```python
from build123d import *

# Parameters (mm, degrees)
SKETCH_1_R          = 4
EXTRUDE_1_DEPTH     = 3
EXTRUDE_2_DEPTH     = 3
SKETCH_3_W          = 36.5
SKETCH_3_H          = 5.8
SKETCH_3_R          = 0.65
EXTRUDE_3_DEPTH     = 1.75
SKETCH_3_4_R        = 1
CUT_EXTRUDE_1_DEPTH = 1.2
EXTRUDE_START       = -22
SKETCH_3_5_W        = 36.5
SKETCH_3_5_H        = 5.8
SKETCH_3_5_R        = 0.65
EXTRUDE_4_DEPTH     = 1.75
CUT_EXTRUDE_START   = -20.8
SKETCH_3_6_R        = 1
CUT_EXTRUDE_2_DEPTH = 1.2
SKETCH_5_R          = 0.4
CUT_EXTRUDE_3_DEPTH = 2


with BuildPart() as part:
    # 草图1 → 凸台-拉伸1 (new body)
    with BuildSketch(Plane(origin=(0, 0, 0), x_dir=(0, 0, -1), z_dir=(1, 0, 0))):
        with BuildLine():
            ThreePointArc((-13.5, 3.1e-08), (-11.998004256, -6.188529216), (-7.826237921, -11))
            Line((-7.826237921, -11), (7.826237921, -11))
            ThreePointArc((7.826237921, -11), (11.998004249, -6.18852923), (13.5, 0))
            ThreePointArc((13.5, 0), (11.998004249, 6.18852923), (7.826237921, 11))
            Line((7.826237921, 11), (-7.826237921, 11))
            ThreePointArc((-7.826237921, 11), (-11.998004242, 6.188529244), (-13.5, 3.1e-08))
        make_face()
        Circle(SKETCH_1_R, mode=Mode.SUBTRACT)
    extrude(amount=EXTRUDE_1_DEPTH)

    # 草图2 → 凸台-拉伸2 (add)
    with BuildSketch(Plane(origin=(3, 0, 0), x_dir=(0, 0, -1), z_dir=(1, 0, 0))):
        with BuildLine():
            ThreePointArc((-5.159699604, 11), (-6.577220881, 10.215804691), (-7.877816956, 9.25))
            Line((-7.877816956, 9.25), (7.877816956, 9.25))
            ThreePointArc((7.877816956, 9.25), (6.577220881, 10.215804691), (5.159699604, 11))
            Line((5.159699604, 11), (-5.159699604, 11))
        make_face()
        with BuildLine():
            Line((-9.83298022, 9.25), (-7.877816956, 9.25))
            ThreePointArc((-7.877816956, 9.25), (-6.577220881, 10.215804691), (-5.159699604, 11))
            Line((-5.159699604, 11), (-7.826237921, 11))
            ThreePointArc((-7.826237921, 11), (-8.87285869, 10.174594767), (-9.83298022, 9.25))
        make_face()
        with BuildLine():
            Line((-12.15, 5.884513574), (-12.15, 2.4e-08))
            ThreePointArc((-12.15, 2.4e-08), (-11.030366626, 5.09445896), (-7.877816956, 9.25))
            Line((-7.877816956, 9.25), (-9.83298022, 9.25))
            ThreePointArc((-9.83298022, 9.25), (-11.119553928, 7.65542425), (-12.15, 5.884513574))
        make_face()
        with BuildLine():
            ThreePointArc((-12.15, 5.884513574), (-13.5, 0), (-12.15, -5.884513574))
            Line((-12.15, -5.884513574), (-12.15, 2.4e-08))
            Line((-12.15, 2.4e-08), (-12.15, 5.884513574))
        make_face()
        with BuildLine():
            ThreePointArc((-12.15, -5.884513574), (-11.119553928, -7.65542425), (-9.83298022, -9.25))
            Line((-9.83298022, -9.25), (-7.877816956, -9.25))
            ThreePointArc((-7.877816956, -9.25), (-11.030366636, -5.094458939), (-12.15, 2.4e-08))
            Line((-12.15, 2.4e-08), (-12.15, -5.884513574))
        make_face()
        with BuildLine():
            Line((-7.877816956, -9.25), (-9.83298022, -9.25))
            ThreePointArc((-9.83298022, -9.25), (-8.87285869, -10.174594767), (-7.826237921, -11))
            Line((-7.826237921, -11), (-5.159699604, -11))
            ThreePointArc((-5.159699604, -11), (-6.577220881, -10.215804691), (-7.877816956, -9.25))
        make_face()
        with BuildLine():
            Line((7.877816956, -9.25), (-7.877816956, -9.25))
            ThreePointArc((-7.877816956, -9.25), (-6.577220881, -10.215804691), (-5.159699604, -11))
            Line((-5.159699604, -11), (5.159699604, -11))
            ThreePointArc((5.159699604, -11), (6.577220881, -10.215804691), (7.877816956, -9.25))
        make_face()
        with BuildLine():
            Line((9.83298022, -9.25), (7.877816956, -9.25))
            ThreePointArc((7.877816956, -9.25), (6.577220881, -10.215804691), (5.159699604, -11))
            Line((5.159699604, -11), (7.826237921, -11))
            ThreePointArc((7.826237921, -11), (8.87285869, -10.174594767), (9.83298022, -9.25))
        make_face()
        with BuildLine():
            ThreePointArc((12.15, 0), (11.030366631, -5.09445895), (7.877816956, -9.25))
            Line((7.877816956, -9.25), (9.83298022, -9.25))
            ThreePointArc((9.83298022, -9.25), (11.119553928, -7.65542425), (12.15, -5.884513574))
            Line((12.15, -5.884513574), (12.15, 0))
        make_face()
        with BuildLine():
            Line((12.15, 5.884513574), (12.15, 0))
            Line((12.15, 0), (12.15, -5.884513574))
            ThreePointArc((12.15, -5.884513574), (13.5, 0), (12.15, 5.884513574))
        make_face()
        with BuildLine():
            ThreePointArc((7.877816956, 9.25), (11.030366631, 5.09445895), (12.15, 0))
            Line((12.15, 0), (12.15, 5.884513574))
            ThreePointArc((12.15, 5.884513574), (11.119553928, 7.65542425), (9.83298022, 9.25))
            Line((9.83298022, 9.25), (7.877816956, 9.25))
        make_face()
        with BuildLine():
            ThreePointArc((5.159699604, 11), (6.577220881, 10.215804691), (7.877816956, 9.25))
            Line((7.877816956, 9.25), (9.83298022, 9.25))
            ThreePointArc((9.83298022, 9.25), (8.87285869, 10.174594767), (7.826237921, 11))
            Line((7.826237921, 11), (5.159699604, 11))
        make_face()
    extrude(amount=EXTRUDE_2_DEPTH)

    # 草图3 → 凸台-拉伸3 (add)
    with BuildSketch(Plane(origin=(0, 11, 0), x_dir=(1, 0, 0), z_dir=(0, 1, 0))):
        with Locations((18.25, 0)):
            Rectangle(SKETCH_3_W, SKETCH_3_H)
        with Locations(Location((35, 0, 0), (0, 0, 270))):
            Circle(SKETCH_3_R, mode=Mode.SUBTRACT)
    extrude(amount=-EXTRUDE_3_DEPTH)

    # 草图3<4> → 切除-拉伸1 (cut)
    with BuildSketch(Plane(origin=(0, 11, 0), x_dir=(1, 0, 0), z_dir=(0, 1, 0))):
        with Locations(Location((35, 0, 0), (0, 0, 270))):
            Circle(SKETCH_3_4_R)
    extrude(amount=-CUT_EXTRUDE_1_DEPTH, mode=Mode.SUBTRACT)

    # 草图3<5> → 凸台-拉伸4 (add)
    with BuildSketch(Plane(origin=(0, 11, 0), x_dir=(1, 0, 0), z_dir=(0, 1, 0)).offset(EXTRUDE_START)):
        with Locations((18.25, 0)):
            Rectangle(SKETCH_3_5_W, SKETCH_3_5_H)
        with Locations(Location((35, 0, 0), (0, 0, 270))):
            Circle(SKETCH_3_5_R, mode=Mode.SUBTRACT)
    extrude(amount=EXTRUDE_4_DEPTH)

    # 草图3<6> → 切除-拉伸2 (cut)
    with BuildSketch(Plane(origin=(0, 11, 0), x_dir=(1, 0, 0), z_dir=(0, 1, 0)).offset(CUT_EXTRUDE_START)):
        with Locations(Location((35, 0, 0), (0, 0, 270))):
            Circle(SKETCH_3_6_R)
    extrude(amount=-CUT_EXTRUDE_2_DEPTH, mode=Mode.SUBTRACT)

    # 草图5 → 切除-拉伸3 (cut)
    with BuildSketch(Plane(origin=(0, 11, 0), x_dir=(1, 0, 0), z_dir=(0, 1, 0))):
        with Locations(Location((1.5, -4.695742753, 0), (0, 0, 270))):
            Circle(SKETCH_5_R)
        with Locations(Location((1.5, 4.695742753, 0), (0, 0, 270))):
            Circle(SKETCH_5_R)
    extrude(amount=-CUT_EXTRUDE_3_DEPTH, mode=Mode.SUBTRACT)


solid = part.part
```
Verification items for the finished model (mm, model axes). A direction names the side the tool comes from. Give positions to 0.01 mm unless a question says otherwise; leave off trailing zeros. Write each loop counter-clockwise with the first axis right and the second up, starting at its lowest first coordinate (ties: lowest second). Pieces come first, ordered by that corner, then holes. Notation, with made-up numbers: (71, 22) - (111, 22) arc R28 cw to (111, 59) - close; hole circle Ø6 at (58, 70.25). An arc over 180 degrees is marked (long way). Put each result on its own line as item: value.
Q1. Section check B-B on x = 35. Record the cut outline in (y, z), and give its area (3 significant figures).
Result:
outline: (-11, -2.9) - (-9.25, -2.9) - (-9.25, -0.65) - (-9.8, -0.65) - (-9.8, -1) - (-11, -1) - close; (-11, 1) - (-9.8, 1) - (-9.8, 0.65) - (-9.25, 0.65) - (-9.25, 2.9) - (-11, 2.9) - close; (9.25, -2.9) - (11, -2.9) - (11, -1) - (9.8, -1) - (9.8, -0.65) - (9.25, -0.65) - close; (9.25, 0.65) - (9.8, 0.65) - (9.8, 1) - (11, 1) - (11, 2.9) - (9.25, 2.9) - close
area: 14.1 mm2
Q2. Set-up check for faces 5 (the face through (6, 0, 13)), 6 (the face through (16, -9.25, 0)), 7 (the face through (6, 0.1, -12.5)), 8 (the face through (1.257, 10.014, -5.013)): record each of +Z, -Z, +X, -X, +Y, -Y from which the full face is reachable in a straight line by a thin tool's end or side.
Result:
face 5: +Z, +X, +Y, -Y
face 6: +X
face 7: -Z, +X, +Y, -Y
face 8: +Y
Q3. Scan lines: probe 1 along Y at (x, z) = (9.5, -2.5); probe 2 along Y at (x, z) = (1.3, 0); probe 3 along Z at (x, y) = (35, 9.4). Record each from-to range of solid material in increasing order. Write a range as from..to.
Result:
probe 1: -11..-9.25, 9.25..11
probe 2: -11..-4, 4..11
probe 3: -2.9..-0.65, 0.65..2.9
Q4. Section check C-C on y = 1.5. Record the cut outline in (x, z).
Result:
outline: (0, -13.42) - (6, -13.42) - (6, -12.06) - (3, -12.06) - (3, -3.71) - (0, -3.71) - close; (0, 3.71) - (3, 3.71) - (3, 12.06) - (6, 12.06) - (6, 13.42) - (0, 13.42) - close
Q5. Mould release check, pull along Z, two halves, no side actions. Record for faces 1 (the face through (34.365, 9.529, -0.141)), 2 (the face through (34.365, -9.529, -0.141)), 3 (the face through (21, -10, -2.9)), 4 (the face through (36.5, 10, 0)): released by +Z, released by -Z, zero draft, split by the parting line, or undercut.
Result:
face 1: undercut
face 2: undercut
face 3: released by -Z
face 4: zero draft
Q6. Section check A-A on z = 0. Record the cut outline in (x, y).
Result:
outline: (0, -11) - (34, -11) - (34, -9.8) - (34.35, -9.8) - (34.35, -9.25) - (3, -9.25) - (3, -4) - (0, -4) - close; (0, 4) - (3, 4) - (3, 9.25) - (34.35, 9.25) - (34.35, 9.8) - (34, 9.8) - (34, 11) - (0, 11) - close; (35.65, -9.8) - (36, -9.8) - (36, -11) - (36.5, -11) - (36.5, -9.25) - (35.65, -9.25) - close; (35.65, 9.25) - (36.5, 9.25) - (36.5, 11) - (36, 11) - (36, 9.8) - (35.65, 9.8) - close
Q7. Depth check by flat-ended pin: P1, Ø0.5, axis at x = 18, y = -10, coming from the +Z side; P2, Ø5, axis at y = -1, z = -6, coming from the +X side; P3, Ø1.8, axis at x = 35, z = 0, coming from the -Y side; P4, Ø2.5, axis at x = 35, z = 0, coming from the -Y side. Enter the tip coordinate at first touch or a pass-through.
Result:
P1: z = 2.9
P2: x = 3
P3: y = -9.8
P4: y = -11
Q8. Section check D-D on x = 24.5. Record the cut outline in (y, z), and give its area (3 significant figures).
Result:
outline: (-11, -2.9) - (-9.25, -2.9) - (-9.25, 2.9) - (-11, 2.9) - close; (9.25, -2.9) - (11, -2.9) - (11, 2.9) - (9.25, 2.9) - close
area: 20.3 mm2
